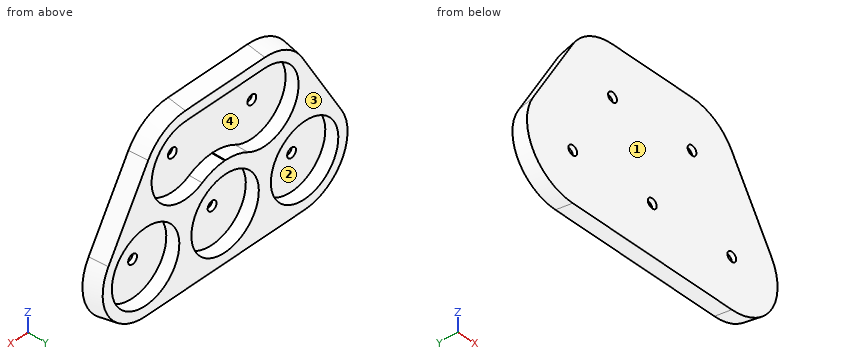
```python
from build123d import *

# Parameters (mm, degrees)
BOSS_EXTRUDE1_DEPTH = 4
BOSS_EXTRUDE1_TAPER = 10
CUT_EXTRUDE1_START  = 4
SKETCH1_3_R         = 1.1
CUT_EXTRUDE1_DEPTH  = 4
CUT_EXTRUDE2_START  = 4
SKETCH1_4_R         = 8.4
SKETCH1_4_R_2       = 1.1
CUT_EXTRUDE2_DEPTH  = 3


with BuildPart() as part:
    # Sketch1 → Boss-Extrude1 (new body)
    with BuildSketch(Plane(origin=(0, 0, 0), x_dir=(1, 0, 0), z_dir=(0, 1, 0))):
        with BuildLine():
            Line((-49.472689603, -5.7), (-39.572689603, -22.847302995))
            ThreePointArc((-39.572689603, -22.847302995), (-35.4, -27.019992598), (-29.7, -28.547302995))
            Line((-29.7, -28.547302995), (-9.9, -28.547302995))
            ThreePointArc((-9.9, -28.547302995), (-4.2, -27.019992598), (-0.027310397, -22.847302995))
            Line((-0.027310397, -22.847302995), (9.872689603, -5.7))
            ThreePointArc((9.872689603, -5.7), (9.872689603, 5.7), (0, 11.4))
            Line((0, 11.4), (-39.6, 11.4))
            ThreePointArc((-39.6, 11.4), (-49.472689603, 5.7), (-49.472689603, -5.7))
        make_face()
    extrude(amount=BOSS_EXTRUDE1_DEPTH, taper=BOSS_EXTRUDE1_TAPER)

    # Sketch1<3> → Cut-Extrude1 (cut)
    with BuildSketch(Plane(origin=(0, 0, 0), x_dir=(1, 0, 0), z_dir=(0, 1, 0)).offset(CUT_EXTRUDE1_START)):
        with Locations(Location((-9.9, -17.147302995, 0), (0, 0, 270))):
            Circle(SKETCH1_3_R)
        with Locations(Location((-19.8, 0, 0), (0, 0, 270))):
            Circle(SKETCH1_3_R)
        with Locations(Location((0, 0, 0), (0, 0, 270))):
            Circle(SKETCH1_3_R)
        with Locations(Location((-29.7, -17.147302995, 0), (0, 0, 270))):
            Circle(SKETCH1_3_R)
        with Locations(Location((-39.6, 0, 0), (0, 0, 270))):
            Circle(SKETCH1_3_R)
    extrude(amount=-CUT_EXTRUDE1_DEPTH, mode=Mode.SUBTRACT)

    # Sketch1<4> → Cut-Extrude2 (cut)
    # profile 1 of 4: a face of its own
    with BuildSketch(Plane(origin=(0, 0, 0), x_dir=(1, 0, 0), z_dir=(0, 1, 0)).offset(CUT_EXTRUDE2_START)):
        with Locations(Location((0, 0, 0), (0, 0, 270))):
            Circle(SKETCH1_4_R)
        with Locations(Location((0, 0, 0), (0, 0, 270))):
            Circle(SKETCH1_4_R_2, mode=Mode.SUBTRACT)
    # profile 2 of 4: a face of its own
    with BuildSketch(Plane(origin=(0, 0, 0), x_dir=(1, 0, 0), z_dir=(0, 1, 0)).offset(CUT_EXTRUDE2_START)):
        with BuildLine():
            Line((-29.7, -25.547302995), (-9.9, -25.547302995))
            ThreePointArc((-9.9, -25.547302995), (-1.786223222, -14.97322241), (-14.100001087, -9.872690231))
            ThreePointArc((-14.100001087, -9.872690231), (-16.822981756, -11.004424673), (-19.745150662, -11.39986805))
            ThreePointArc((-19.745150662, -11.39986805), (-19.772689603, -11.447302995), (-19.8, -11.494869891))
            ThreePointArc((-19.8, -11.494869891), (-19.827310397, -11.447302995), (-19.854849338, -11.39986805))
            ThreePointArc((-19.854849338, -11.39986805), (-22.777018876, -11.004424502), (-25.500000049, -9.872689575))
            ThreePointArc((-25.500000049, -9.872689575), (-37.813776948, -14.973223043), (-29.7, -25.547302995))
        make_face()
        with Locations(Location((-9.9, -17.147302995, 0), (0, 0, 270))):
            Circle(SKETCH1_4_R_2, mode=Mode.SUBTRACT)
        with Locations(Location((-29.7, -17.147302995, 0), (0, 0, 270))):
            Circle(SKETCH1_4_R_2, mode=Mode.SUBTRACT)
    # profile 3 of 4: a face of its own
    with BuildSketch(Plane(origin=(0, 0, 0), x_dir=(1, 0, 0), z_dir=(0, 1, 0)).offset(CUT_EXTRUDE2_START)):
        with Locations(Location((-19.8, 0, 0), (0, 0, 270))):
            Circle(SKETCH1_4_R)
        with Locations(Location((-19.8, 0, 0), (0, 0, 270))):
            Circle(SKETCH1_4_R_2, mode=Mode.SUBTRACT)
    # profile 4 of 4: a face of its own
    with BuildSketch(Plane(origin=(0, 0, 0), x_dir=(1, 0, 0), z_dir=(0, 1, 0)).offset(CUT_EXTRUDE2_START)):
        with Locations(Location((-39.6, 0, 0), (0, 0, 270))):
            Circle(SKETCH1_4_R)
        with Locations(Location((-39.6, 0, 0), (0, 0, 270))):
            Circle(SKETCH1_4_R_2, mode=Mode.SUBTRACT)
    extrude(amount=-CUT_EXTRUDE2_DEPTH, mode=Mode.SUBTRACT)


solid = part.part
```
Geometry check sheet. Reference: the model listing, model coordinates, mm. Face numbers are marked on the shaded views. A direction names the side the tool comes from. Give positions to 0.01 mm unless a question says otherwise; leave off trailing zeros. Write item = value, one per line. Start each with the question number.
1) Gauge pin test, flat ends, axial feed: pin 1 Ø8.5 at (x, z) = (-14, 15) entering from +Y; pin 2 Ø1 at (y, z) = (1.5, 3.5) entering from +X; pin 3 Ø1 at (y, z) = (0.5, -6) entering from -X. Record the tip position at first contact, or that the pin passes through.
2) Draft check along Z on the marked faces 3 and 4. Enter one of: released by +Z, released by -Z, zero draft, split by the parting line, or undercut.
3) Section check A-A (z = 0). Count the separate pieces of the cut face and the enclosed holes in it, then the cut area to 3 significant figures.
4) Access from +Z, -Z, +X, -X, +Y, -Y to the whole of each face (thin tool, end or side, straight path). Record for the marked faces 1 and 2.
5) Scan lines: L1, parallel to Z at x = -25, y = 1.4; L2, parallel to X at y = 3.35, z = 0; L3, parallel to X at y = 2.8, z = 0. Record each from-to range of solid material in increasing order.
Geometry check:
q1.pin_1 = 1
q1.pin_2 = 10.75
q1.pin_3 = -49.5
q2.face_3 = zero draft
q2.face_4 = undercut
q3.separate_pieces = 4
q3.enclosed_holes = 0
q3.area = 89.0 mm2
q4.face_1 = +Z, -Z, +X, -X, -Y
q4.face_2 = +Y
q5.L1 = -11.15 to -6.6, 6.6 to 10.14, 25.55 to 28.3
q5.L2 = -50.41 to -48, -31.2 to -28.2, -11.4 to -8.4, 8.4 to 10.81
q5.L3 = -50.51 to -48, -31.2 to -28.2, -11.4 to -8.4, 8.4 to 10.91
